from build123d import *

# Parameters (mm, degrees)
BOSS_EXTRUDE7_DEPTH        = 4
CUT_EXTRUDE1_DEPTH         = 4
CUT_EXTRUDE5_SCIECIA_DEPTH = 4


with BuildPart() as part:
    # Sweep1: sweep along a path in Sketch2path
    with BuildLine(Plane.XY) as sweep1_path:
        Line((40.002617842, -0.001745558), (30.002617994, -2.28e-07))
        ThreePointArc((30.002617994, -2.28e-07), (30.001308997, -5.7e-08), (30, 0))
        Line((30, 0), (0, 0))
    # Sketch3 → Sweep1 (sweep)
    with BuildSketch(Plane(origin=(0, 0, 0), x_dir=(0, 0, -1), z_dir=(1, 0, 0))):
        with BuildLine():
            Line((-16.65, -4), (-16.65, 4))
            ThreePointArc((-16.65, 4), (-15.478427125, 6.828427125), (-12.65, 8))
            Line((-12.65, 8), (12.65, 8))
            ThreePointArc((12.65, 8), (15.478427125, 6.828427125), (16.65, 4))
            Line((16.65, 4), (16.65, -4))
            ThreePointArc((16.65, -4), (15.478427125, -6.828427125), (12.65, -8))
            Line((12.65, -8), (-12.65, -8))
            ThreePointArc((-12.65, -8), (-15.478427125, -6.828427125), (-16.65, -4))
        make_face()
        with BuildLine():
            Line((-15.65, -4), (-15.65, 4))
            ThreePointArc((-15.65, 4), (-14.771320344, 6.121320344), (-12.65, 7))
            Line((-12.65, 7), (12.65, 7))
            ThreePointArc((12.65, 7), (14.771320344, 6.121320344), (15.65, 4))
            Line((15.65, 4), (15.65, -4))
            ThreePointArc((15.65, -4), (14.771320344, -6.121320344), (12.65, -7))
            Line((12.65, -7), (-12.65, -7))
            ThreePointArc((-12.65, -7), (-14.771320344, -6.121320344), (-15.65, -4))
        make_face(mode=Mode.SUBTRACT)
    sweep(path=sweep1_path.line)

    # Sketch14 → Boss-Extrude7 (add, symmetric)
    with BuildSketch(Plane.ZY):
        with BuildLine():
            Line((-15.65, -4), (-15.65, 4))
            ThreePointArc((-15.65, 4), (-14.771320344, 6.121320344), (-12.65, 7))
            Line((-12.65, 7), (12.65, 7))
            ThreePointArc((12.65, 7), (14.771320344, 6.121320344), (15.65, 4))
            Line((15.65, 4), (15.65, -4))
            ThreePointArc((15.65, -4), (14.771320344, -6.121320344), (12.65, -7))
            Line((12.65, -7), (-12.65, -7))
            ThreePointArc((-12.65, -7), (-14.771320344, -6.121320344), (-15.65, -4))
        make_face()
        with BuildLine():
            Line((-12.65, 5.8), (12.65, 5.8))
            ThreePointArc((12.65, 5.8), (13.922792206, 5.272792206), (14.45, 4))
            Line((14.45, 4), (14.45, -4))
            ThreePointArc((14.45, -4), (13.922792206, -5.272792206), (12.65, -5.8))
            Line((12.65, -5.8), (-12.65, -5.8))
            ThreePointArc((-12.65, -5.8), (-13.922792206, -5.272792206), (-14.45, -4))
            Line((-14.45, -4), (-14.45, 4))
            ThreePointArc((-14.45, 4), (-13.922792206, 5.272792206), (-12.65, 5.8))
        make_face(mode=Mode.SUBTRACT)
    extrude(amount=BOSS_EXTRUDE7_DEPTH, both=True)

    # Sketch15 → Cut-Extrude1 (cut)
    with BuildSketch(Plane.ZY.offset(4)):
        with BuildLine():
            Line((-12.65, -7), (12.65, -7))
            ThreePointArc((12.65, -7), (14.771320344, -6.121320344), (15.65, -4))
            Line((15.65, -4), (15.65, 4))
            ThreePointArc((15.65, 4), (14.771320344, 6.121320344), (12.65, 7))
            Line((12.65, 7), (-12.65, 7))
            ThreePointArc((-12.65, 7), (-14.771320344, 6.121320344), (-15.65, 4))
            Line((-15.65, 4), (-15.65, -4))
            ThreePointArc((-15.65, -4), (-14.771320344, -6.121320344), (-12.65, -7))
        make_face()
        with BuildLine():
            Line((-15.45, 4), (-15.45, -4))
            ThreePointArc((-15.45, -4), (-14.629898987, -5.979898987), (-12.65, -6.8))
            Line((-12.65, -6.8), (12.65, -6.8))
            ThreePointArc((12.65, -6.8), (14.629898987, -5.979898987), (15.45, -4))
            Line((15.45, -4), (15.45, 4))
            ThreePointArc((15.45, 4), (14.629898987, 5.979898987), (12.65, 6.8))
            Line((12.65, 6.8), (-12.65, 6.8))
            ThreePointArc((-12.65, 6.8), (-14.629898987, 5.979898987), (-15.45, 4))
        make_face(mode=Mode.SUBTRACT)
    extrude(amount=-CUT_EXTRUDE1_DEPTH, mode=Mode.SUBTRACT)

    # Sketch20 → Cut-Extrude5 sciecia (cut)
    with BuildSketch(Plane.ZY.offset(4)):
        with BuildLine():
            Line((16.65, 2.715147186), (16.65, 4))
            ThreePointArc((16.65, 4), (15.478427125, 6.828427125), (12.65, 8))
            Line((12.65, 8), (11.365147186, 8))
            Line((11.365147186, 8), (16.65, 2.715147186))
        make_face()
        with BuildLine():
            Line((-11.365147186, 8), (-12.65, 8))
            ThreePointArc((-12.65, 8), (-15.478427125, 6.828427125), (-16.65, 4))
            Line((-16.65, 4), (-16.65, 2.715147186))
            Line((-16.65, 2.715147186), (-11.365147186, 8))
        make_face()
        with BuildLine():
            Line((11.365147186, -8), (12.65, -8))
            ThreePointArc((12.65, -8), (15.478427125, -6.828427125), (16.65, -4))
            Line((16.65, -4), (16.65, -2.715147186))
            Line((16.65, -2.715147186), (11.365147186, -8))
        make_face()
        with BuildLine():
            Line((-16.65, -2.715147186), (-16.65, -4))
            ThreePointArc((-16.65, -4), (-15.478427125, -6.828427125), (-12.65, -8))
            Line((-12.65, -8), (-11.365147186, -8))
            Line((-11.365147186, -8), (-16.65, -2.715147186))
        make_face()
    extrude(amount=-CUT_EXTRUDE5_SCIECIA_DEPTH, mode=Mode.SUBTRACT)


solid = part.part
Work out the finished part from the listing and answer in its coordinate system (mm). A direction names the side the tool comes from. Round coordinates to 2 decimals unless told otherwise and drop trailing zeros. Loops run counter-clockwise (first coordinate to the right, second up) from the corner with the lowest first, then second, coordinate; pieces in that order, holes last. Notation, with made-up numbers: (3, -26.75) - (61, -26.75) arc R14 ccw to (61, -14.75) - close; hole circle Ø3 at (-34.75, -33.75). An arc over 180 degrees is marked (long way). One line per item, written item: value.
Q1. Straight lines are drawn through the part: probe 1 along Y at (x, z) = (13.5, -7); probe 2 along Z at (x, y) = (38, -3.5); probe 3 along Z at (x, y) = (-1, -0.5). For each, find the intervals that lie inside material, in ascending order.
Check values:
probe 1: -8 to -7, 7 to 8
probe 2: -16.65 to -15.65, 15.65 to 16.65
probe 3: -15.45 to -14.45, 14.45 to 15.45
Q2. Find section A-A on x = 19.5. Give the vertices of the cut face in (y, z).
Check values:
outline: (-8, -12.65) arc R4 ccw to (-4, -16.65) - (4, -16.65) arc R4 ccw to (8, -12.65) - (8, 12.65) arc R4 ccw to (4, 16.65) - (-4, 16.65) arc R4 ccw to (-8, 12.65) - close; hole (-7, -12.65) arc R3 ccw to (-4, -15.65) - (4, -15.65) arc R3 ccw to (7, -12.65) - (7, 12.65) arc R3 ccw to (4, 15.65) - (-4, 15.65) arc R3 ccw to (-7, 12.65) - close
Q3. For faces 4 (the flat face through (-2, 0, 15.45)), 5 (the cylindrical face through (-0.056, -5.016, 14.136)), 6 (the flat face through (4, -6, 0)), determine the directions among +Z, -Z, +X, -X, +Y, -Y from which every point of the face is accessible in a straight line to the end or side of a thin tool.
Check values:
face 4: +Z, -X, +Y, -Y
face 5: +X, -X
face 6: +X
Q4. Each of these flat-tipped pins is pushed along its axis until it touches: pin 1 Ø3 at (x, y) = (-2.5, -1) entering from +Z; pin 2 Ø1.2 at (x, z) = (-3, 6) entering from -Y. Where does it stop, or does it pass through?
Check values:
pin 1: z = 15.45
pin 2: y = -6.8
Q5. The mould has two halves that part along Y. Classify faces 1 (the flat face through (0, 0, -14.45)), 2 (the cylindrical face through (14.79, 6.859, -15.447)), 3 (the flat face through (0, 7, -3)): +Y half, -Y half, draft (parallel to the pull), parting line (faces both ways), or undercut.
Check values:
face 1: undercut
face 2: +Y half
face 3: draft
Q6. Find section C-C on y = -3. Give the vertices of the cut face in (x, z).
Check values:
outline: (-4, -15.45) - (0, -15.45) - (0, -16.65) - (40, -16.65) - (40, -15.65) - (4, -15.65) - (4, -14.45) - (-4, -14.45) - close; (-4, 14.45) - (4, 14.45) - (4, 15.65) - (40, 15.65) - (40, 16.65) - (0, 16.65) - (0, 15.45) - (-4, 15.45) - close
Q7. Find section D-D on x = 2. Give the vertices of the cut face in (y, z).
Check values:
outline: (-8, -12.65) arc R4 ccw to (-4, -16.65) - (4, -16.65) arc R4 ccw to (8, -12.65) - (8, 12.65) arc R4 ccw to (4, 16.65) - (-4, 16.65) arc R4 ccw to (-8, 12.65) - close; hole (-5.8, -12.65) arc R1.8 ccw to (-4, -14.45) - (4, -14.45) arc R1.8 ccw to (5.8, -12.65) - (5.8, 12.65) arc R1.8 ccw to (4, 14.45) - (-4, 14.45) arc R1.8 ccw to (-5.8, 12.65) - close
